Autodesk Inventor part; units mm, degrees
ref_plane "YZ Plane" through (0, 0, 0) normal (1, 0, 0) x (0, 1, 0)
ref_plane "XZ Plane" through (0, 0, 0) normal (0, 1, 0) x (-1, 0, 0)
ref_plane "XY Plane" through (0, 0, 0) normal (0, 0, 1) x (1, 0, 0)
sketch "Эскиз1" plane through (0, 0, 0) normal (0, 1, 0) x (-1, 0, 0)
  circle A0 centre (12.55, 18.8) radius 1.25
  circle A1 centre (-12.55, 18.8) radius 1.25
  circle A2 centre (-12.55, -18.8) radius 1.25
  circle A3 centre (12.55, -18.8) radius 1.25
  circle A4 centre (15, -15) radius 1.5
  circle A5 centre (15, 15) radius 1.5
  circle A6 centre (10, 10) radius 1.5
  circle A7 centre (10, -10) radius 1.5
  circle A8 centre (-10, 10) radius 1.5
  circle A9 centre (-10, -10) radius 1.5
  circle A10 centre (-15, -15) radius 1.5
  circle A11 centre (-15, 15) radius 1.5
  arc A12 (16.7678, 13.2322) -> (17.1011, 16.3547) centre (15, 15) ccw
  arc A13 (-16.7678, -13.2322) -> (-17.1011, -16.3547) centre (-15, -15) ccw
  arc A14 (17.1011, -16.3547) -> (16.7678, -13.2322) centre (15, -15) ccw
  arc A15 (-17.1011, 16.3547) -> (-16.7678, 13.2322) centre (-15, 15) ccw
  line L0 (16.7678, -13.2322) -> (7.0711, -3.5355)
  line L1 (-3.5355, 7.0711) -> (-5.9595, 9.4951)
  line L2 (-5.9595, -9.4951) -> (-3.5355, -7.0711)
  line L3 (7.0711, 3.5355) -> (16.7678, 13.2322)
  line L4 (5.9595, 9.4951) -> (3.5355, 7.0711)
  line L5 (-7.0711, -3.5355) -> (-16.7678, -13.2322)
  line L6 (-16.7678, 13.2322) -> (-7.0711, 3.5355)
  line L7 (3.5355, -7.0711) -> (5.9595, -9.4951)
  line L8 (10.1488, 19.4958) -> (8.4933, 13.7829)
  arc A16 (14.6511, 20.1547) -> (10.1488, 19.4958) centre (12.55, 18.8) ccw
  line L9 (10, -10) -> (12.55, -18.8) construction
  line L10 (8.4933, -13.7829) -> (10.1488, -19.4958)
  arc A17 (10.1488, -19.4958) -> (14.6511, -20.1547) centre (12.55, -18.8) ccw
  line L11 (-10.1488, -19.4958) -> (-8.4933, -13.7829)
  arc A18 (-14.6511, -20.1547) -> (-10.1488, -19.4958) centre (-12.55, -18.8) ccw
  line L12 (-8.4933, 13.7829) -> (-10.1488, 19.4958)
  arc A19 (-10.1488, 19.4958) -> (-14.6511, 20.1547) centre (-12.55, 18.8) ccw
  line L13 (10, 10) -> (10.4175, 11.4407) construction
  line L14 (12.2021, 17.5994) -> (12.55, 18.8) construction
  line L15 (12.55, 18.8) -> (15, 15) construction
  line L16 (17.1011, 16.3547) -> (14.6511, 20.1547)
  arc A20 (14.6511, 20.1547) -> (10.1488, 19.4958) centre (12.55, 18.8) ccw
  arc A21 (16.7678, 13.2322) -> (17.1011, 16.3547) centre (15, 15) ccw
  line L17 (15, -15) -> (12.55, -18.8) construction
  line L18 (11.8055, -15.3411) -> (11.6276, -15.617)
  line L19 (14.6511, -20.1547) -> (17.1011, -16.3547)
  arc A22 (17.1011, -16.3547) -> (16.7678, -13.2322) centre (15, -15) ccw
  arc A23 (10.1488, -19.4958) -> (14.6511, -20.1547) centre (12.55, -18.8) ccw
  line L20 (-12.55, -18.8) -> (-15, -15) construction
  line L21 (-17.1011, -16.3547) -> (-14.6511, -20.1547)
  arc A24 (-14.6511, -20.1547) -> (-10.1488, -19.4958) centre (-12.55, -18.8) ccw
  arc A25 (-16.7678, -13.2322) -> (-17.1011, -16.3547) centre (-15, -15) ccw
  line L22 (-15, 15) -> (-12.55, 18.8) construction
  line L23 (-14.6511, 20.1547) -> (-17.1011, 16.3547)
  arc A26 (-17.1011, 16.3547) -> (-16.7678, 13.2322) centre (-15, 15) ccw
  arc A27 (-10.1488, 19.4958) -> (-14.6511, 20.1547) centre (-12.55, 18.8) ccw
  arc A28 (7.0711, 3.5355) -> (7.0711, -3.5355) centre (10.6066, 0) ccw
  arc A29 (-3.5355, 7.0711) -> (3.5355, 7.0711) centre (0, 10.6066) ccw
  arc A30 (3.5355, -7.0711) -> (-3.5355, -7.0711) centre (0, -10.6066) ccw
  arc A31 (-7.0711, -3.5355) -> (-7.0711, 3.5355) centre (-10.6066, 0) ccw
  arc A32 (5.9595, 9.4951) -> (8.4933, 13.7829) centre (-1.1115, 16.5661) ccw
  arc A33 (-8.4933, 13.7829) -> (-5.9595, 9.4951) centre (1.1115, 16.5661) ccw
  arc A34 (-5.9595, -9.4951) -> (-8.4933, -13.7829) centre (1.1115, -16.5661) ccw
  arc A35 (8.4933, -13.7829) -> (5.9595, -9.4951) centre (-1.1115, -16.5661) ccw
  point P0 (0, 0)
  point P1 (0, 0)
  point P2 (0, 0)
  point P3 (11.275, 14.4)
  point P4 (11.275, -14.4)
  point P5 (-11.275, -14.4)
  point P6 (-11.275, 14.4)
  point P7 (13.775, 16.9)
  point P8 (13.775, -16.9)
  point P9 (-13.775, -16.9)
  point P10 (-13.775, 16.9)
  dimension "d12" = 3
  dimension "d7" = 2.5
  dimension "d8" = 2.5
  dimension "d9" = 2.5
  dimension "d10" = 3
  dimension "d11" = 3
  dimension "d13" = 3
  dimension "d14" = 3
  dimension "d15" = 3
  dimension "d16" = 3
  dimension "d17" = 3
  dimension "d21" = 5
  dimension "d24" = 5
  dimension "d25" = 5
  dimension "d26" = 5
  dimension "d27" = 5
  dimension "d28" = 5
  dimension "d29" = 10
extrude "Выдавливание1" add sketch "Эскиз1" along normal blind 2
properties part number "2030fermto"
Verification items for the finished model (mm, model axes). A direction names the side the tool comes from. Round coordinates to 2 decimals unless told otherwise and drop trailing zeros. Order: outer loops, then holes, each group sorted by start corner. A loop starts at its lowest first (then second) coordinate and runs counter-clockwise, first axis right, second up. Notation, with made-up numbers: (60, 44) - (89, 44) arc R20 cw to (89, 53) - close; hole circle Ø1 at (73, -40). An arc over 180 degrees is marked (long way). Use CSV: the item, a comma, the result in double quotes.
(1) Thickness scan on probe 1 along Z at (x, y) = (12.55, 0.8); probe 2 along Z at (x, y) = (-15, 1.2); probe 3 along X at (y, z) = (0.4, -18). Record the ranges inside material, lowest first. Write a range as from..to.
Entries:
probe 1,"-21.3..-20.05, -17.55..-9.01, 9.01..17.55, 20.05..21.3"
probe 2,"-19.61..-16.5, -13.5..-11.46, 11.46..13.5, 16.5..19.61"
probe 3,"-16.04..-13.51, -11.59..-9.72, 9.72..11.59, 13.51..16.04"
(2) Section check D-D on y = 0.75. State how many separate pieces and enclosed holes the cut face has, and give its area (3 significant figures).
Entries:
separate pieces,"1"
enclosed holes,"12"
area,"514 mm^2"
(3) Gauge pin test, flat end, axial feed: pin 1 Ø2.5 at (x, z) = (-10, -10) entering from +Y. Record the tip position at first contact, or that the pin passes through.
Entries:
pin 1,"through"
(4) Section check A-A on z = 10. Record the boundary of the cut face in (x, y), and give its area (3 significant figures).
Entries:
outline,"(-13.54, 0) - (-11.5, 0) - (-11.5, 2) - (-13.54, 2) - close; (-8.5, 0) - (-6.43, 0) - (-6.43, 2) - (-8.5, 2) - close; (6.43, 0) - (8.5, 0) - (8.5, 2) - (6.43, 2) - close; (11.5, 0) - (13.54, 0) - (13.54, 2) - (11.5, 2) - close"
area,"16.4 mm^2"
(5) Mould release check, pull along Z, two halves, no side actions. Record for faces 4 (the face through (-8.8, 1, -9.1)), 5 (the face through (-12.23, 0.99, -21.28)), 6 (the face through (-7.515, 0.986, 11.509)): released by +Z, released by -Z, zero draft, split by the parting line, or undercut.
Entries:
face 4,"undercut"
face 5,"released by -Z"
face 6,"released by +Z"
(6) Section check C-C on z = -17. Record the boundary of the cut face in (x, y), and give its area (3 significant figures).
Entries:
outline,"(-16.69, 0) - (-9.43, 0) - (-9.43, 2) - (-16.69, 2) - close; (9.43, 0) - (16.69, 0) - (16.69, 2) - (9.43, 2) - close"
area,"29.0 mm^2"
(7) Access from +Z, -Z, +X, -X, +Y, -Y to the whole of each face (thin tool, end or side, straight path). Record for faces 1 (the face through (9.333, 0.986, -16.679)), 2 (the face through (11.852, 0.986, -8.316)), 3 (the face through (-11.852, 0.986, 8.316)).
Entries:
face 1,"-Z, +Y, -Y"
face 2,"+X, +Y, -Y"
face 3,"-X, +Y, -Y"
(8) Section check B-B on x = -12.5. Record the boundary of the cut face in (y, z), and give its area (3 significant figures).
Entries:
outline,"(0, -21.3) - (2, -21.3) - (2, -20.05) - (0, -20.05) - close; (0, -17.55) - (2, -17.55) - (2, -8.96) - (0, -8.96) - close; (0, 8.96) - (2, 8.96) - (2, 17.55) - (0, 17.55) - close; (0, 20.05) - (2, 20.05) - (2, 21.3) - (0, 21.3) - close"
area,"39.3 mm^2"
